For this review, take the finished solid that the model builds, in its own axes (mm). A direction names the side the tool comes from. Round coordinates to 2 decimals unless told otherwise and drop trailing zeros. Loops run counter-clockwise (first coordinate to the right, second up) from the corner with the lowest first, then second, coordinate; pieces in that order, holes last. Notation, with made-up numbers: (47, -11.5) -> (89, -11.5) arc R3 cw to (89, -6.5) -> close; hole circle Ø10 at (-20, 70.25). An arc over 180 degrees is marked (long way). Write each question's results on one line, items separated by ' | '.
```python
from build123d import *

# Parameters (mm, degrees)
SKETCH1_W           = 20
SKETCH1_H           = 20
SKETCH1_W_2         = 17
SKETCH1_H_2         = 17
BOSS_EXTRUDE1_DEPTH = 300
SKETCH2_R           = 2.125
CUT_EXTRUDE1_DEPTH  = 301.83217913


with BuildPart() as part:
    # Sketch1 → Boss-Extrude1 (new body)
    with BuildSketch(Plane.XY):
        Rectangle(SKETCH1_W, SKETCH1_H)
        Rectangle(SKETCH1_W_2, SKETCH1_H_2, mode=Mode.SUBTRACT)
    extrude(amount=-BOSS_EXTRUDE1_DEPTH)

    # Sketch2 → Cut-Extrude1 (cut, through all)
    with BuildSketch(Plane(origin=(0, 10, 0), x_dir=(1, 0, 0), z_dir=(0, 1, 0))):
        with Locations(Location((0, 10, 0), (0, 0, 270))):
            Circle(SKETCH2_R)
        with Locations(Location((0, 80, 0), (0, 0, 270))):
            Circle(SKETCH2_R)
        with Locations(Location((0, 150, 0), (0, 0, 270))):
            Circle(SKETCH2_R)
        with Locations(Location((0, 220, 0), (0, 0, 270))):
            Circle(SKETCH2_R)
        with Locations(Location((0, 290, 0), (0, 0, 270))):
            Circle(SKETCH2_R)
        with Locations(Location((0, 195, 0), (0, 0, 270))):
            Circle(SKETCH2_R)
        with Locations(Location((0, 105, 0), (0, 0, 90))):
            Circle(SKETCH2_R)
    extrude(amount=-CUT_EXTRUDE1_DEPTH, mode=Mode.SUBTRACT)


solid = part.part
```
1. Consider section C-C (z = -280). State the section outline as (x, y) points, plus the area to 3 significant figures.
Values found:
outline: (-10, -10) -> (10, -10) -> (10, 10) -> (-10, 10) -> close; hole (-8.5, -8.5) -> (8.5, -8.5) -> (8.5, 8.5) -> (-8.5, 8.5) -> close | area: 111 mm2
2. Consider section A-A (x = -5). State the section outline as (y, z) points.
Values found:
outline: (-10, -300) -> (-8.5, -300) -> (-8.5, 0) -> (-10, 0) -> close; (8.5, -300) -> (10, -300) -> (10, 0) -> (8.5, 0) -> close
3. To check wall thickness, follow probe 1 along X at (y, z) = (-9.2, -10) (3 decimals); probe 2 along Y at (x, z) = (4.5, -162). State the ranges of each line that lie inside material, in increasing order.
Values found:
probe 1: x = -10 to -2.125, 2.125 to 10 | probe 2: y = -10 to -8.5, 8.5 to 10
4. Tool access review of faces 4 (the face through (-10, 0, -148)), 5 (the face through (-2, 8.5, -148)): name each direction out of +Z, -Z, +X, -X, +Y, -Y from which nothing blocks a thin tool from reaching the whole face with its end or side.
Values found:
face 4: +Z, -Z, -X, +Y, -Y | face 5: +Z, -Z
5. For pin 1 (5 mm diameter, centred on x = 0, z = -105, fed in from -Y); pin 2 (3 mm diameter, centred on x = -2.5, y = 6.5, fed in from +Z), all flat-tipped, find the tip position at first contact; note any pin that passes through.
Values found:
pin 1: stops at y = -10 | pin 2: passes through
6. Draft analysis for pull direction Y (two halves, no side actions). For faces 1 (the face through (-8.5, 0, -148)), 2 (the face through (2, 10, -148)), 3 (the face through (-9, 0, -300)), state which applies: released by +Y, released by -Y, zero draft, split by the parting line, or undercut.
Values found:
face 1: undercut | face 2: released by +Y | face 3: zero draft
